```python
from build123d import *

# Parameters (mm, degrees)
REVOLUTION_ANGLE = 250


with BuildPart() as part:
    # Sketch → Revolution (revolve)
    with BuildSketch(Plane.YZ):
        Polygon((-75, 22.5), (0, 22.5), (0, 55), (-35, 55), (-35, 77.5), (-70, 77.5), (-70, 100), (-105, 100), (-105, 80), (-88, 80), (-88, 57.5), (-55, 57.5), (-55, 32.5), (-75, 32.5), align=None)
    revolve(axis=Axis((0, 0, 0), (0, 1, 0)), revolution_arc=REVOLUTION_ANGLE)


solid = part.part
```
Geometry check sheet. Reference: the model listing, model coordinates, mm. A direction names the side the tool comes from. Round coordinates to 2 decimals unless told otherwise and drop trailing zeros. Order: outer loops, then holes, each group sorted by start corner. A loop starts at its lowest first (then second) coordinate and runs counter-clockwise, first axis right, second up. Notation, with made-up numbers: M 54,60.5 L 90,60.5 A20 cw 90,82.5 Z; hole C 65,56.5 d9. An arc over 180 degrees is marked long. Answer as CSV lines item,"result".
1) Tool access check on faces 1 (the face through (83.63, -87.74, -54.83)), 2 (the face through (75, -70, -22)), 3 (the face through (61, -105, -52)), 4 (the face through (0, -53, 53)), 5 (the face through (48.086, -71.269, -31.527)). Record the directions out of +Z, -Z, +X, -X, +Y, -Y that give a thin tool (end or side, any length) a straight path to the whole face; none if there is none.
Entries:
face 1,"+Y, -Y"
face 2,"+Y"
face 3,"+Z, -Z, +X, -X, -Y"
face 4,"+Z, -X, +Y, -Y"
face 5,"-Y"
2) Thickness scan on probe 1 along X at (y, z) = (-72, 0); probe 2 along Y at (x, z) = (33.5, 13); probe 3 along X at (y, z) = (-74, 19). Record the ranges inside material, lowest first. Write a range as [from, to].
Entries:
probe 1,"[22.5, 32.5], [57.5, 100]"
probe 2,"[-55, 0]"
probe 3,"[12.05, 26.37], [54.27, 98.18]"
3) Sectioned sample at A-A on z = 0. Record the cut outline in (x, y).
Entries:
outline,"M 22.5,-75 L 32.5,-75 L 32.5,-55 L 57.5,-55 L 57.5,-88 L 80,-88 L 80,-105 L 100,-105 L 100,-70 L 77.5,-70 L 77.5,-35 L 55,-35 L 55,0 L 22.5,0 Z"
4) Sectioned sample at D-D on z = 70. Record the cut outline in (x, y), and give its area (3 significant figures).
Entries:
outline,"M 0,-88 L 38.73,-88 L 38.73,-105 L 71.41,-105 L 71.41,-70 L 33.26,-70 L 33.26,-35 L 0,-35 Z"
area,"3,010 mm2"
5) Gauge pin test, flat ends, axial feed: pin 1 Ø5 at (x, z) = (70.5, -20) entering from -Y; pin 2 Ø5 at (y, z) = (-59.5, 73.5) entering from +X; pin 3 Ø4 at (x, y) = (42.5, -71) entering from +Z. Record the tip position at first contact, or that the pin passes through.
Entries:
pin 1,"y = -88"
pin 2,"x = 31.07"
pin 3,"z = 91.43"
6) Mould release check, pull along Z, two halves, no side actions. Record for faces 6 (the face through (26, 0, -11)), 7 (the face through (27, -55, -26)), 8 (the face through (-50, -53.2, -18.2)): +Z half, -Z half, draft (parallel to the pull), parting line (faces both ways), or undercut.
Entries:
face 6,"draft"
face 7,"undercut"
face 8,"+Z half"
7) Sectioned sample at B-B on x = 17. Record the cut outline in (y, z).
Entries:
outline,"M -105,-98.54 L -70,-98.54 L -70,-75.61 L -35,-75.61 L -35,-52.31 L 0,-52.31 L 0,-14.74 L -75,-14.74 L -75,-27.7 L -55,-27.7 L -55,-54.93 L -88,-54.93 L -88,-78.17 L -105,-78.17 Z; M -105,78.17 L -88,78.17 L -88,54.93 L -55,54.93 L -55,27.7 L -75,27.7 L -75,14.74 L 0,14.74 L 0,52.31 L -35,52.31 L -35,75.61 L -70,75.61 L -70,98.54 L -105,98.54 Z"
8) Sectioned sample at C-C on y = -97. Record the cut outline in (x, z).
Entries:
outline,"M -93.97,-34.2 A100 ccw long 0,100 L 0,80 A80 cw long -75.18,-27.36 Z"
